```python
from build123d import *

# Parameters (mm, degrees)
SKETCH_2_W          = 41
SKETCH_2_H          = 106
SKETCH_2_R          = 1.65
EXTRUDE_3_DEPTH     = 17
SKETCH_5_R          = 1.65
CUT_EXTRUDE_2_DEPTH = 112.094554322
SKETCH_6_W          = 41
SKETCH_6_H          = 106
EXTRUDE_4_DEPTH     = 3
CUT_EXTRUDE_START   = -2
SKETCH_7_W          = 10.5
SKETCH_7_H          = 10.5
SKETCH_7_W_2        = 10
SKETCH_7_H_2        = 10
CUT_EXTRUDE_3_DEPTH = 110.593010534
SKETCH_9_W          = 1.5
SKETCH_9_H          = 9
CUT_EXTRUDE_4_DEPTH = 112.593010534
SKETCH_10_R         = 3.5
CUT_EXTRUDE_7_DEPTH = 112.094554322
SKETCH_12_W         = 20
SKETCH_12_H         = 3
CUT_EXTRUDE_8_DEPTH = 16
CUT_EXTRUDE_9_DEPTH = 112.094554322
FILLET_1_R          = 3.1
FILLET_2_R          = 3.1
FILLET_3_R          = 3.1
FILLET_4_R          = 8


with BuildPart() as part:
    # 草图2 → 凸台-拉伸3 (new body)
    with BuildSketch(Plane.XY):
        with Locations((17.5, 50)):
            Rectangle(SKETCH_2_W, SKETCH_2_H)
        Polygon((9, 0), (9, 9), (0, 9), (0, 91), (9, 91), (9, 100), (26, 100), (26, 91), (35, 91), (35, 9), (26, 9), (26, 0), align=None, mode=Mode.SUBTRACT)
        with Locations((4.5, 4.5)):
            Circle(SKETCH_2_R, mode=Mode.SUBTRACT)
        with Locations((4.5, 95.5)):
            Circle(SKETCH_2_R, mode=Mode.SUBTRACT)
        with Locations((30.5, 95.5)):
            Circle(SKETCH_2_R, mode=Mode.SUBTRACT)
    extrude(amount=EXTRUDE_3_DEPTH)

    # 草图5 → 切除-拉伸2 (cut, through all)
    with BuildSketch(Plane.XY.offset(17)):
        with Locations((30.5, 4.5)):
            Circle(SKETCH_5_R)
    extrude(amount=-CUT_EXTRUDE_2_DEPTH, mode=Mode.SUBTRACT)

    # 草图6 → 凸台-拉伸4 (add)
    with BuildSketch(Plane(origin=(0, 0, 0), x_dir=(-1, 0, 0), z_dir=(0, 0, -1))):
        with Locations((-17.5, 50)):
            Rectangle(SKETCH_6_W, SKETCH_6_H)
    extrude(amount=EXTRUDE_4_DEPTH)

    # 草图7 → 切除-拉伸3 (cut, through all)
    with BuildSketch(Plane.XY.offset(17).offset(CUT_EXTRUDE_START)):
        with Locations((2.25, 97.75)):
            Rectangle(SKETCH_7_W, SKETCH_7_H)
        with Locations((33, 98)):
            Rectangle(SKETCH_7_W_2, SKETCH_7_H_2)
        with Locations((2.25, 2.25)):
            Rectangle(SKETCH_7_W, SKETCH_7_H)
        with Locations((32.75, 2.25)):
            Rectangle(SKETCH_7_W, SKETCH_7_H)
    extrude(amount=-CUT_EXTRUDE_3_DEPTH, mode=Mode.SUBTRACT)

    # 草图9 → 切除-拉伸4 (cut, through all)
    with BuildSketch(Plane.XY.offset(17)):
        with Locations((8.25, 4.5)):
            Rectangle(SKETCH_9_W, SKETCH_9_H)
        with Locations((26.75, 4.5)):
            Rectangle(SKETCH_9_W, SKETCH_9_H)
    extrude(amount=-CUT_EXTRUDE_4_DEPTH, mode=Mode.SUBTRACT)

    # 草图10 → 切除-拉伸7 (cut, through all)
    with BuildSketch(Plane.XY):
        with Locations((28.5, 83.63)):
            Circle(SKETCH_10_R)
    extrude(amount=-CUT_EXTRUDE_7_DEPTH, mode=Mode.SUBTRACT)

    # 草图12 → 切除-拉伸8 (cut)
    with BuildSketch(Plane(origin=(0, 0, -3), x_dir=(-1, 0, 0), z_dir=(0, 0, -1))):
        with Locations((-17.5, -1.5)):
            Rectangle(SKETCH_12_W, SKETCH_12_H)
    extrude(amount=-CUT_EXTRUDE_8_DEPTH, mode=Mode.SUBTRACT)

    # 草图13 → 切除-拉伸9 (cut, through all)
    with BuildSketch(Plane.XY):
        Polygon((0, 49), (0, 9), (9, 9), (9, 0), (26, 0), (26, 9), (35, 9), (35, 61), (26, 61), (26, 49), align=None)
    extrude(amount=-CUT_EXTRUDE_9_DEPTH, mode=Mode.SUBTRACT)

    # 圆角1
    # the kernel refuses this fillet: 3.1 mm, written as the material it takes off along each edge
    with BuildSketch(Plane(origin=(-3, 100.25, -3), x_dir=(0, 0, 1), z_dir=(0, -1, 0))) as fillet_1_piece_1:
        with BuildLine():
            CenterArc((FILLET_1_R, -FILLET_1_R), FILLET_1_R, 90, 90)
            Line((0, -FILLET_1_R), (0, 0))
            Line((0, 0), (FILLET_1_R, 0))
        make_face()
    extrude(amount=100.5, mode=Mode.SUBTRACT)
    with BuildSketch(Plane(origin=(38, -0.25, -3), x_dir=(0, 0, 1), z_dir=(0, 1, 0))) as fillet_1_piece_2:
        with BuildLine():
            CenterArc((FILLET_1_R, -FILLET_1_R), FILLET_1_R, 90, 90)
            Line((0, -FILLET_1_R), (0, 0))
            Line((0, 0), (FILLET_1_R, 0))
        make_face()
    extrude(amount=101, mode=Mode.SUBTRACT)

    # 圆角2
    # the kernel refuses this fillet: 3.1 mm, written as the material it adds along each edge
    with BuildSketch(Plane(origin=(7.5, -3, 15), x_dir=(-1, 0, 0), z_dir=(0, 1, 0))) as fillet_2_piece_1:
        with BuildLine():
            CenterArc((2.898275349, -3.1), FILLET_2_R, 90, 69.216440404)
            Line((0, -2), (0, 0))
            Line((0, 0), (2.898275349, 0))
        make_face()
    extrude(amount=3)
    with BuildSketch(Plane(origin=(27.5, -3, 15), x_dir=(0, 0, -1), z_dir=(0, 1, 0))) as fillet_2_piece_2:
        with BuildLine():
            CenterArc((3.1, -2.898275349), FILLET_2_R, 110.783559596, 69.216440404)
            Line((0, -2.898275349), (0, 0))
            Line((0, 0), (2, 0))
        make_face()
    extrude(amount=3)
    with BuildSketch(Plane(origin=(28, 93, 15), x_dir=(0, 1, 0), z_dir=(0, 0, -1))) as fillet_2_piece_3:
        with BuildLine():
            CenterArc((FILLET_2_R, FILLET_2_R), FILLET_2_R, 180, 90)
            Line((0, FILLET_2_R), (0, 0))
            Line((0, 0), (FILLET_2_R, 0))
        make_face()
    extrude(amount=18)
    with BuildSketch(Plane(origin=(7.5, 92.5, 22.75), x_dir=(-1, 0, 0), z_dir=(0, 0, -1))) as fillet_2_piece_4_section:
        with BuildLine():
            CenterArc((FILLET_2_R, FILLET_2_R), FILLET_2_R, 180, 90)
            Line((0, FILLET_2_R), (0, 0))
            Line((0, 0), (FILLET_2_R, 0))
        make_face()
    fillet_2_piece_4 = extrude(amount=25.75, mode=Mode.PRIVATE)
    fillet_2_piece_4 = split(fillet_2_piece_4, bisect_by=Plane(origin=(6.807559389, 93.192440611, 17), z_dir=(0, 0, -1)), keep=Keep.TOP, mode=Mode.PRIVATE)
    add(fillet_2_piece_4)

    # 圆角3
    # the kernel refuses this fillet: 3.1 mm, written as the material it takes off along each edge
    with BuildSketch(Plane(origin=(10.6, 99.9, 0.1), x_dir=(0, 0, -1), z_dir=(0, 1, 0))) as fillet_3_piece_1_section:
        Polygon((0, 0), (FILLET_3_R * 1.02, 0), (FILLET_3_R * 1.02, FILLET_3_R * 1.02), (0, FILLET_3_R * 1.02), align=None)
    fillet_3_piece_1 = extrude(amount=FILLET_3_R * 1.02, mode=Mode.PRIVATE)
    fillet_3_piece_1 = fillet_3_piece_1 - Plane(origin=(10.6, 99.9, 0.1), x_dir=(0.7071067811865475, 0, 0.7071067811865475), z_dir=(0, 1, 0)) * Sphere(FILLET_3_R, mode=Mode.PRIVATE)
    add(fillet_3_piece_1, mode=Mode.SUBTRACT)
    with BuildSketch(Plane(origin=(24.9, 99.9, 0.1), x_dir=(1, 0, 0), z_dir=(0, 1, 0))) as fillet_3_piece_2_section:
        Polygon((0, 0), (FILLET_3_R * 1.02, 0), (FILLET_3_R * 1.02, FILLET_3_R * 1.02), (0, FILLET_3_R * 1.02), align=None)
    fillet_3_piece_2 = extrude(amount=FILLET_3_R * 1.02, mode=Mode.PRIVATE)
    fillet_3_piece_2 = fillet_3_piece_2 - Plane(origin=(24.9, 99.9, 0.1), x_dir=(-0.7071067811865475, 0, 0.7071067811865475), z_dir=(0, 1, 0)) * Sphere(FILLET_3_R, mode=Mode.PRIVATE)
    add(fillet_3_piece_2, mode=Mode.SUBTRACT)
    with BuildSketch(Plane(origin=(7.5, 99.9, -3), x_dir=(1, 0, 0), z_dir=(0, -1, 0))) as fillet_3_piece_3:
        with BuildLine():
            CenterArc((FILLET_3_R, FILLET_3_R), FILLET_3_R, 180, 90)
            Line((0, FILLET_3_R), (0, 0))
            Line((0, 0), (FILLET_3_R, 0))
        make_face()
    extrude(amount=4.3, mode=Mode.SUBTRACT)
    with BuildSketch(Plane(origin=(4.4, 95.6, -3), x_dir=(1, 0, 0), z_dir=(0, 1, 0))) as fillet_3_piece_4:
        with BuildLine():
            CenterArc((3.1 + FILLET_3_R, -FILLET_3_R), FILLET_3_R, 90, 90)
            Line((3.1, -FILLET_3_R), (3.1, 0))
            Line((3.1, 0), (3.1 + FILLET_3_R, 0))
        make_face()
    revolve(axis=Axis((4.4, 95.6, -3), (0, 0, -1)), revolution_arc=90, mode=Mode.SUBTRACT)
    with BuildSketch(Plane(origin=(4.4, 92.5, -3), x_dir=(0, 0, 1), z_dir=(-1, 0, 0))) as fillet_3_piece_5:
        with BuildLine():
            CenterArc((FILLET_3_R, -FILLET_3_R), FILLET_3_R, 90, 90)
            Line((0, -FILLET_3_R), (0, 0))
            Line((0, 0), (FILLET_3_R, 0))
        make_face()
    extrude(amount=4.3, mode=Mode.SUBTRACT)
    with BuildSketch(Plane(origin=(0.1, 92.5, 0.1), x_dir=(0, 0, -1), z_dir=(1, 0, 0))) as fillet_3_piece_6:
        with BuildLine():
            CenterArc((3.1 - FILLET_3_R, -FILLET_3_R), FILLET_3_R, 0, 90)
            Line((3.1, -FILLET_3_R), (3.1, 0))
            Line((3.1, 0), (3.1 - FILLET_3_R, 0))
        make_face()
    revolve(axis=Axis((0.1, 92.5, 0.1), (0, 1, 0)), revolution_arc=90, mode=Mode.SUBTRACT)
    with BuildSketch(Plane(origin=(28, 99.9, -3), x_dir=(0, 0, 1), z_dir=(0, -1, 0))) as fillet_3_piece_7:
        with BuildLine():
            CenterArc((FILLET_3_R, FILLET_3_R), FILLET_3_R, 180, 90)
            Line((0, FILLET_3_R), (0, 0))
            Line((0, 0), (FILLET_3_R, 0))
        make_face()
    extrude(amount=3.8, mode=Mode.SUBTRACT)
    with BuildSketch(Plane(origin=(31.1, 96.1, -3), x_dir=(0, -1, 0), z_dir=(1, 0, 0))) as fillet_3_piece_8:
        with BuildLine():
            CenterArc((3.1 + FILLET_3_R, -FILLET_3_R), FILLET_3_R, 90, 90)
            Line((3.1, -FILLET_3_R), (3.1, 0))
            Line((3.1, 0), (3.1 + FILLET_3_R, 0))
        make_face()
    revolve(axis=Axis((31.1, 96.1, -3), (0, 0, -1)), revolution_arc=90, mode=Mode.SUBTRACT)
    with BuildSketch(Plane(origin=(31.1, 93, -3), x_dir=(0, -1, 0), z_dir=(1, 0, 0))) as fillet_3_piece_9:
        with BuildLine():
            CenterArc((FILLET_3_R, -FILLET_3_R), FILLET_3_R, 90, 90)
            Line((0, -FILLET_3_R), (0, 0))
            Line((0, 0), (FILLET_3_R, 0))
        make_face()
    extrude(amount=3.8, mode=Mode.SUBTRACT)
    with BuildSketch(Plane(origin=(34.9, 93, 0.1), x_dir=(0, 0, -1), z_dir=(-1, 0, 0))) as fillet_3_piece_10:
        with BuildLine():
            CenterArc((3.1 - FILLET_3_R, FILLET_3_R), FILLET_3_R, 270, 90)
            Line((3.1 - FILLET_3_R, 0), (3.1, 0))
            Line((3.1, 0), (3.1, FILLET_3_R))
        make_face()
    revolve(axis=Axis((34.9, 93, 0.1), (0, -1, 0)), revolution_arc=90, mode=Mode.SUBTRACT)
    with BuildSketch(Plane(origin=(28, 103, 15), x_dir=(-1, 0, 0), z_dir=(0, 0, -1)), Plane(origin=(-3, 92.5, 15), x_dir=(0, -1, 0), z_dir=(0, 0, -1))) as fillet_3_piece_11:
        with BuildLine():
            CenterArc((FILLET_3_R, -FILLET_3_R), FILLET_3_R, 90, 90)
            Line((0, -FILLET_3_R), (0, 0))
            Line((0, 0), (FILLET_3_R, 0))
        make_face()
    extrude(amount=14.9, mode=Mode.SUBTRACT)
    with BuildSketch(Plane(origin=(7.5, 103, 15), x_dir=(1, 0, 0), z_dir=(0, 0, -1)), Plane(origin=(38, 93, 15), x_dir=(0, -1, 0), z_dir=(0, 0, -1))) as fillet_3_piece_12:
        with BuildLine():
            CenterArc((FILLET_3_R, FILLET_3_R), FILLET_3_R, 180, 90)
            Line((0, FILLET_3_R), (0, 0))
            Line((0, 0), (FILLET_3_R, 0))
        make_face()
    extrude(amount=14.9, mode=Mode.SUBTRACT)
    with BuildSketch(Plane(origin=(24.9, 103, -3), x_dir=(0, 0, 1), z_dir=(-1, 0, 0))) as fillet_3_piece_13:
        with BuildLine():
            CenterArc((FILLET_3_R, -FILLET_3_R), FILLET_3_R, 90, 90)
            Line((0, -FILLET_3_R), (0, 0))
            Line((0, 0), (FILLET_3_R, 0))
        make_face()
    extrude(amount=14.3, mode=Mode.SUBTRACT)
    with BuildSketch(Plane(origin=(-3, 7.5, 15), x_dir=(0, 1, 0), z_dir=(0, 0, -1))) as fillet_3_piece_14:
        with BuildLine():
            CenterArc((FILLET_3_R, FILLET_3_R), FILLET_3_R, 180, 90)
            Line((0, FILLET_3_R), (0, 0))
            Line((0, 0), (FILLET_3_R, 0))
        make_face()
    extrude(amount=22.65, mode=Mode.SUBTRACT)
    with BuildSketch(Plane(origin=(38, 7.5, 15), x_dir=(0, 1, 0), z_dir=(0, 0, -1))) as fillet_3_piece_15:
        with BuildLine():
            CenterArc((FILLET_3_R, -FILLET_3_R), FILLET_3_R, 90, 90)
            Line((0, -FILLET_3_R), (0, 0))
            Line((0, 0), (FILLET_3_R, 0))
        make_face()
    extrude(amount=22.65, mode=Mode.SUBTRACT)

    # 圆角4
    fillet_4_edges = [part.edges().sort_by_distance(p)[0] for p in [
        (-3, 103, 16),
        (38, 103, 16),
        (38, -3, 16),
        (-3, -3, 16),
    ]]
    fillet(fillet_4_edges, radius=FILLET_4_R)


solid = part.part
```
Design review of the part built by this model. Coordinates are the model's own, in mm. A direction names the side the tool comes from. Coordinates: 2 decimals unless noted, no trailing zeros. Loops run counter-clockwise (first coordinate to the right, second up) from the corner with the lowest first, then second, coordinate; pieces in that order, holes last.
Q1. Tool access review of faces 1 (the face through (27.5, 8, 11)), 2 (the face through (-2.116, 91.568, 7.654)), 3 (the face through (2, 4, 15)): name each direction out of +Z, -Z, +X, -X, +Y, -Y from which nothing blocks a thin tool from reaching the whole face with its end or side.
Reported:
face 1: +Z, -Z
face 2: -Z, -X, +Y
face 3: -Z, -X
Q2. For pin 1 (3 mm diameter, centred on x = 34.5, y = 1, fed in from -Z); pin 2 (8 mm diameter, centred on x = 31.5, z = 4.5, fed in from -Y); pin 3 (1.1 mm diameter, centred on y = 98, z = 9, fed in from +X), all flat-tipped, find the tip position at first contact; note any pin that passes through.
Reported:
pin 1: stops at z = 15
pin 2: stops at y = 7.5
pin 3: stops at x = 28
Q3. To check wall thickness, follow line 1 (Y direction, x = 4.5, z = 16.5); line 2 (Y direction, x = 34.5, z = 4.75); line 3 (X direction, y = 29.5, z = 14.5). State the ranges of each line that lie inside material, in increasing order.
Reported:
line 1: y = -2.98 to 2.85, 6.15 to 9, 91 to 93.85, 97.15 to 102.98
line 2: y = 7.5 to 9, 91 to 93
line 3: x = -3 to 0, 35 to 38
Q4. We need section B-B on x = 20. State the section outline as (y, z) points, and give its area (3 significant figures).
Reported:
outline: (-3, 13) - (0, 13) - (0, 17) - (-3, 17) - close; (49, -3) - (99.9, -3) arc R3.1 ccw to (103, 0.1) - (103, 17) - (100, 17) - (100, 0) - (49, 0) - close
area: 223 mm2
Q5. We need section A-A on y = 83.63. State the section outline as (x, z) points, and give its area (3 significant figures).
Reported:
outline: (-3, 0.1) arc R3.1 ccw to (0.1, -3) - (25, -3) - (25, 0) - (0, 0) - (0, 17) - (-3, 17) - close; (32, -3) - (34.9, -3) arc R3.1 ccw to (38, 0.1) - (38, 17) - (35, 17) - (35, 0) - (32, 0) - close
area: 200 mm2
Q6. The part is to be moulded in two halves that separate along Y. For faces 4 (the face through (26, 55, -1)), 5 (the face through (2.28, 91.616, -2.068)), 6 (the face through (4, 9, 7)), say which applies: +Y half, -Y half, draft (parallel to the pull), parting line (faces both ways), or undercut.
Reported:
face 4: draft
face 5: +Y half
face 6: undercut
Q7. We need section C-C on z = 5. State the section outline as (x, y) points, and give its area (3 significant figures).
Reported:
outline: (-3, 10.6) arc R3.1 ccw to (0.1, 7.5) - (7.5, 7.5) - (7.5, 9) - (0, 9) - (0, 91) - (9, 91) - (9, 100) - (26, 100) - (26, 91) - (35, 91) - (35, 9) - (27.5, 9) - (27.5, 7.5) - (34.9, 7.5) arc R3.1 ccw to (38, 10.6) - (38, 89.9) arc R3.1 ccw to (34.9, 93) - (31.1, 93) arc R3.1 cw to (28, 96.1) - (28, 99.9) arc R3.1 ccw to (24.9, 103) - (10.6, 103) arc R3.1 ccw to (7.5, 99.9) - (7.5, 95.6) arc R3.1 cw to (4.4, 92.5) - (0.1, 92.5) arc R3.1 ccw to (-3, 89.4) - close
area: 644 mm2
Q8. We need section D-D on y = 64. State the section outline as (x, z) points.
Reported:
outline: (-3, 0.1) arc R3.1 ccw to (0.1, -3) - (34.9, -3) arc R3.1 ccw to (38, 0.1) - (38, 17) - (35, 17) - (35, 0) - (0, 0) - (0, 17) - (-3, 17) - close
